Work out the finished part from the listing and answer in its coordinate system (mm). Face numbers are marked on the shaded views. A direction names the side the tool comes from. Coordinates: 2 decimals unless noted, no trailing zeros. Order: outer loops, then holes, each group sorted by start corner. A loop starts at its lowest first (then second) coordinate and runs counter-clockwise, first axis right, second up. Notation, with made-up numbers: M 25.5,-23 L 51.5,-23 A27 cw 51.5,6 Z; hole C -30,23.5 d1. An arc over 180 degrees is marked long. Answer in a Markdown table with one row per item. Add a question column.
Item 1: The part is cut by section A-A (z = 18). Write down the section's boundary in (x, y).
Item 2: Flat-ended cylindrical pins translate along their axes: pin 1 Ø1.5 at (x, z) = (-20, 8) entering from -Y; pin 2 Ø8 at (y, z) = (-23.5, 12) entering from +X. Find the tip coordinate at first contact, or state that the pin passes through.
Item 3: The part is cut by section D-D (z = 33.5). Write down the section's boundary in (x, y), then the cut area to 3 significant figures.
Item 4: The part is cut by section B-B (x = 21). Write down the section's boundary in (y, z).
Item 5: Consider line 1 (Y direction, x = -9.5, z = 24); line 2 (X direction, y = -16, z = 38); line 3 (X direction, y = -23.5, z = 31). Determine where each line is inside the solid, lowest interval first. Write a range as from..to.
Item 6: The part is cut by section C-C (y = -25). Write down the section's boundary in (x, z), then the cut area to 3 significant figures.
Item 7: Which of the six approach directions +Z, -Z, +X, -X, +Y, -Y give full straight-line access (tool end or side, diameter ignored) to the marked faces 1, 2 and 3?
from build123d import *

# Parameters (mm, degrees)
F1_DEPTH = 40
F2_W     = 10
F2_H     = 20
F3_DEPTH = 10


with BuildPart() as f1:
    # F0 (on Top) → F1 (new body)
    with BuildSketch(Plane.XY):
        Polygon((30, 10), (30, 30), (-30, 30), (-30, -20), (20, -20), (20, 10), align=None)
    extrude(amount=F1_DEPTH)

    # F2 (on face) → F3 (join)
    with BuildSketch(Plane.XZ.offset(20)):
        with Locations((-25, 30)):
            Rectangle(F2_W, F2_H)
    extrude(amount=F3_DEPTH)


solid = f1.part
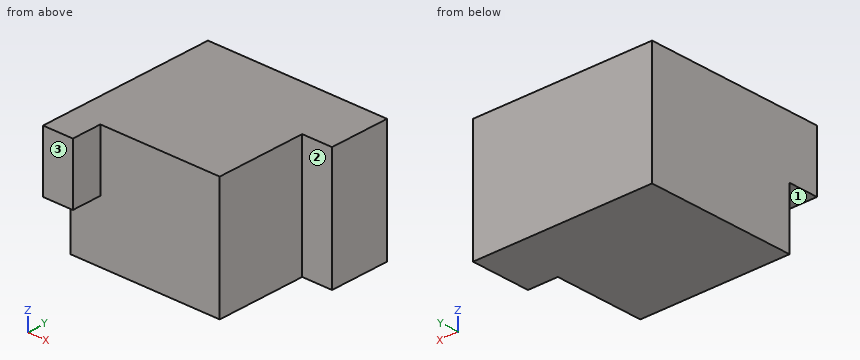
Reply:
| question | item | result |
|---|---|---|
| 1 | outline | M -30,-20 L 20,-20 L 20,10 L 30,10 L 30,30 L -30,30 Z |
| 2 | pin 1 | stops at y = -20 |
| 2 | pin 2 | stops at x = 20 |
| 3 | outline | M -30,-30 L -20,-30 L -20,-20 L 20,-20 L 20,10 L 30,10 L 30,30 L -30,30 Z |
| 3 | area | 2,800 mm2 |
| 4 | outline | M 10,0 L 30,0 L 30,40 L 10,40 Z |
| 5 | line 1 | y = -20..30 |
| 5 | line 2 | x = -30..20 |
| 5 | line 3 | x = -30..-20 |
| 6 | outline | M -30,20 L -20,20 L -20,40 L -30,40 Z |
| 6 | area | 200 mm2 |
| 7 | face 1 | -Z, +X, -X, -Y |
| 7 | face 2 | +Z, -Z, +X, -Y |
| 7 | face 3 | +Z, -Z, +X, -X, -Y |
